```python
from build123d import *

# Parameters (mm, degrees)
ESBO_O1_R                = 4.5
ESBO_O1_R_2              = 1.5
RESSALTO_EXTRUS_O1_DEPTH = 2
RESSALTO_EXTRUS_O2_DEPTH = 18
ESBO_O3_R                = 7
CORTE_EXTRUS_O1_DEPTH    = 18
ESBO_O4_R                = 1.5
CORTE_EXTRUS_O2_DEPTH    = 17


with BuildPart() as part:
    # Esboço1 → Ressalto-extrusão1 (new body)
    with BuildSketch(Plane(origin=(0, 0, 0), x_dir=(1, 0, 0), z_dir=(0, 1, 0))):
        with BuildLine():
            Line((30, 15), (30, 7))
            Line((30, 7), (0, 7))
            Line((0, 7), (0, -7))
            Line((0, -7), (30, -7))
            Line((30, -7), (30, -15))
            Line((30, -15), (-15, -15))
            ThreePointArc((-15, -15), (-30, 0), (-15, 15))
            Line((-15, 15), (30, 15))
        make_face()
        with Locations((-15, 0)):
            Circle(ESBO_O1_R, mode=Mode.SUBTRACT)
        with Locations((-9, -6)):
            Circle(ESBO_O1_R_2, mode=Mode.SUBTRACT)
        with Locations((-6, -8)):
            Circle(ESBO_O1_R_2, mode=Mode.SUBTRACT)
        with Locations((-22, -7)):
            Circle(ESBO_O1_R_2, mode=Mode.SUBTRACT)
        with Locations((-21, 6)):
            Circle(ESBO_O1_R_2, mode=Mode.SUBTRACT)
        with Locations((-24, 8)):
            Circle(ESBO_O1_R_2, mode=Mode.SUBTRACT)
        with Locations((-8, 7)):
            Circle(ESBO_O1_R_2, mode=Mode.SUBTRACT)
    extrude(amount=RESSALTO_EXTRUS_O1_DEPTH)

    # Esboço2 → Ressalto-extrusão2 (add)
    with BuildSketch(Plane(origin=(30, 0, 0), x_dir=(0, 0, -1), z_dir=(1, 0, 0))):
        with BuildLine():
            Line((-15, 2), (-15, 4))
            Line((-15, 4), (-8.61684397, 4))
            ThreePointArc((-8.61684397, 4), (0, 9.5), (8.61684397, 4))
            Line((8.61684397, 4), (15, 4))
            Line((15, 4), (15, 2))
            Line((15, 2), (-15, 2))
        make_face()
    extrude(amount=-RESSALTO_EXTRUS_O2_DEPTH)

    # Esboço3 → Corte-extrusão1 (cut)
    with BuildSketch(Plane(origin=(30, 0, 0), x_dir=(0, 0, -1), z_dir=(1, 0, 0))):
        Circle(ESBO_O3_R)
    extrude(amount=-CORTE_EXTRUS_O1_DEPTH, mode=Mode.SUBTRACT)

    # Esboço4 → Corte-extrusão2 (cut)
    with BuildSketch(Plane(origin=(0, 4, 0), x_dir=(1, 0, 0), z_dir=(0, 1, 0))):
        with Locations((21, 12)):
            Circle(ESBO_O4_R)
        with Locations((21, -12)):
            Circle(ESBO_O4_R)
    extrude(amount=-CORTE_EXTRUS_O2_DEPTH, mode=Mode.SUBTRACT)


solid = part.part
```
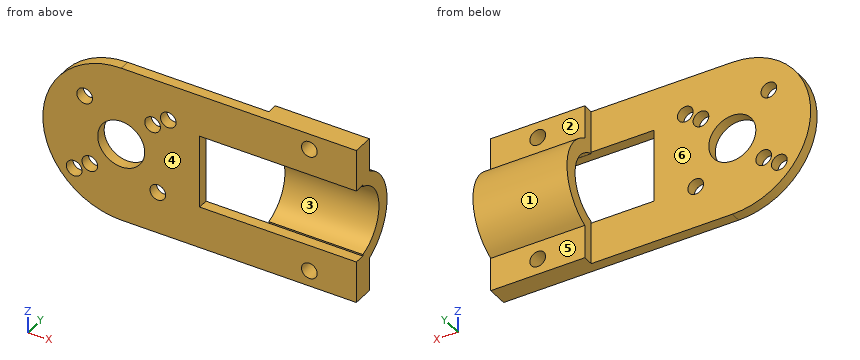
Can you work these out from the model? Positions are in its coordinate system, mm. Face numbers are marked on the shaded views. A direction names the side the tool comes from. Round coordinates to 2 decimals unless told otherwise and drop trailing zeros. Order: outer loops, then holes, each group sorted by start corner. A loop starts at its lowest first (then second) coordinate and runs counter-clockwise, first axis right, second up. Notation, with made-up numbers: (16.25, 12) -> (59.25, 12) arc R20 cw to (59.25, 41) -> close; hole circle Ø5 at (22.25, 39.25). An arc over 180 degrees is marked (long way). Return JSON: item names as keys, results as strings. Group by question number.
1. I need wall thicknesses on line 1 (Z direction, x = -6, y = 0.85); line 2 (X direction, y = 1.55, z = 0); line 3 (X direction, y = 1.25, z = 6). Which ranges of each line are inside material? Lowest first, please. Write a range as [from, to].
2. Which directions (+Z, -Z, +X, -X, +Y, -Y) give clear straight access to the entire face, cutting with the end or side of a thin tool? Please do the marked faces 4, 5 and 6.
3. If we section it at A-A, the plane z = 0: Write out the boundary of the cut face in (x, y).
4. If we section it at D-D, the plane x = 24.5: Write out the boundary of the cut face in (y, z).
5. We'd pull the mould along Z, two halves only. Please class the marked faces 1, 2 and 3: released by +Z, released by -Z, zero draft, split by the parting line, or undercut.
6. If we section it at C-C, the plane y = 6.25: Write out the boundary of the cut face in (x, z), then the cut area to 3 significant figures.
7. Will these pins go through, and if not, where does the flat tip stop? pin 1 (1.9 mm diameter, centred on x = 17, z = 10.5, fed in from +Y); pin 2 (1.8 mm diameter, centred on x = 21, z = -12, fed in from -Y); pin 3 (2 mm diameter, centred on y = 0.5, z = -1.5, fed in from +X); pin 4 (10 mm diameter, centred on x = -22, z = 9, fed in from +Y).
8. If we section it at B-B, the plane z = 12: Write out the boundary of the cut face in (x, y).
Output values:
{
 "1": {"line 1": "[-15, 6.5], [9.5, 15]", "line 2": "[-30, -19.5], [-10.5, 0]", "line 3": "[-28.75, -23.12], [-20.88, -10.5], [-7.5, 0]"},
 "2": {"face 4": "+Z, -Z, +X, -X, -Y", "face 5": "-Z, +X, -X, +Y", "face 6": "+Z, -Z, -X, +Y"},
 "3": {"outline": "(-30, 0) -> (-19.5, 0) -> (-19.5, 2) -> (-30, 2) -> close; (-10.5, 0) -> (0, 0) -> (0, 2) -> (-10.5, 2) -> close; (12, 7) -> (30, 7) -> (30, 9.5) -> (12, 9.5) -> close"},
 "4": {"outline": "(0, -15) -> (4, -15) -> (4, -8.62) arc R9.5 ccw to (4, 8.62) -> (4, 15) -> (0, 15) -> (0, 7) -> (2, 7) -> (2, 6.71) arc R7 cw to (2, -6.71) -> (2, -7) -> (0, -7) -> close"},
 "5": {"face 1": "split by the parting line", "face 2": "zero draft", "face 3": "undercut"},
 "6": {"outline": "(12, -7.15) -> (30, -7.15) -> (30, -3.15) -> (12, -3.15) -> close; (12, 3.15) -> (30, 3.15) -> (30, 7.15) -> (12, 7.15) -> close", "area": "144 mm²"},
 "7": {"pin 1": "y = 4", "pin 2": "through", "pin 3": "x = 0", "pin 4": "y = 2"},
 "8": {"outline": "(-24, 0) -> (19.5, 0) -> (19.5, 4) -> (12, 4) -> (12, 2) -> (-24, 2) -> close; (22.5, 0) -> (30, 0) -> (30, 4) -> (22.5, 4) -> close"}
}
